Source: CAD feature listing. Evaluate the final solid. Frame: model axes, mm. A direction names the side the tool comes from. Give positions to 0.01 mm unless a question says otherwise; leave off trailing zeros. Loops run counter-clockwise (first coordinate to the right, second up) from the corner with the lowest first, then second, coordinate; pieces in that order, holes last. Notation, with made-up numbers: M 53.5,13.5 L 81.5,13.5 A20 cw 81.5,18.5 Z; hole C 40,-4 d4. An arc over 180 degrees is marked long. Write item = value, one per line.
from build123d import *

# Parameters (mm, degrees)
EXTRUDE_1_DEPTH     = 12
SKETCH_2_R          = 6
EXTRUDE_2_DEPTH     = 9
SKETCH_3_R          = 5.25
EXTRUDE_3_DEPTH     = 1
SKETCH_4_R          = 6
EXTRUDE_4_DEPTH     = 2
CHAMFER_1_SIZE      = 0.5
SKETCH_5_R          = 2
CUT_EXTRUDE_1_DEPTH = 5


with BuildPart() as part:
    # 草图1 → 凸台-拉伸1 (new body)
    with BuildSketch(Plane(origin=(0, 0, 0), x_dir=(1, 0, 0), z_dir=(0, 1, 0))):
        with BuildLine():
            Line((-17.5, 6.09769995), (-6.926984364, 18.843732288))
            ThreePointArc((-6.926984364, 18.843732288), (0, 22.09769995), (6.926984364, 18.843732288))
            Line((6.926984364, 18.843732288), (17.5, 6.09769995))
            Line((17.5, 6.09769995), (17.5, 1.09769995))
            Line((17.5, 1.09769995), (-17.5, 1.09769995))
            Line((-17.5, 1.09769995), (-17.5, 6.09769995))
        make_face()
    extrude(amount=EXTRUDE_1_DEPTH)

    # 草图2 → 凸台-拉伸2 (add)
    with BuildSketch(Plane(origin=(0, 0, 0), x_dir=(1, 0, 0), z_dir=(0, 1, 0))):
        with Locations(Location((0, 13.09769995, 0), (0, 0, 270))):
            Circle(SKETCH_2_R)
    extrude(amount=-EXTRUDE_2_DEPTH)

    # 草图3 → 凸台-拉伸3 (add)
    with BuildSketch(Plane(origin=(0, -9, 0), x_dir=(-1, 0, 0), z_dir=(0, -1, 0))):
        with Locations(Location((0, 13.09769995, 0), (0, 0, 270))):
            Circle(SKETCH_3_R)
    extrude(amount=EXTRUDE_3_DEPTH)

    # 草图4 → 凸台-拉伸4 (add)
    with BuildSketch(Plane(origin=(0, -10, 0), x_dir=(-1, 0, 0), z_dir=(0, -1, 0))):
        with Locations(Location((0, 13.09769995, 0), (0, 0, 270))):
            Circle(SKETCH_4_R)
    extrude(amount=EXTRUDE_4_DEPTH)

    # 倒角1
    chamfer_1_edges = [part.edges().sort_by_distance(p)[0] for p in [
        (0, -12, -19.09769995),
    ]]
    chamfer(chamfer_1_edges, length=CHAMFER_1_SIZE)

    # 草图5 → 切除-拉伸1 (cut)
    with BuildSketch(Plane.XY.offset(-1.09769995)):
        with Locations((-10, 6)):
            Circle(SKETCH_5_R)
        with Locations(Location((10, 6, 0), (0, 0, 180))):
            Circle(SKETCH_5_R)
    extrude(amount=-CUT_EXTRUDE_1_DEPTH, mode=Mode.SUBTRACT)


solid = part.part
1. First-contact query: pin 1 Ø5 at (y, z) = (-4.5, -11.5) entering from -X; pin 2 Ø6 at (y, z) = (5.5, -12) entering from +X; pin 3 Ø3.5 at (x, y) = (10, 6) entering from -Z. Flat tips, straight axial feed; report the tip coordinate or a pass-through.
Derived:
pin_1 = -6
pin_2 = 15.09
pin_3 = -17.25
2. Pull-direction query (Y, two-part tool) for faces 5 (the cylindrical face through (11.6, 7.2, -3.6)), 6 (the cylindrical face through (-0.111, 5.916, -22.097)), 7 (the flat face through (0, -12, -13)); classes: +Y half, -Y half, draft (parallel to the pull), parting line (faces both ways), or undercut.
Derived:
face_5 = undercut
face_6 = draft
face_7 = -Y half
3. Cut plane C-C, the plane x = 10. Return the cut outline in (y, z).
Derived:
outline = M 0,-15.14 L 12,-15.14 L 12,-1.1 L 8,-1.1 L 8,-6.1 L 4,-6.1 L 4,-1.1 L 0,-1.1 Z
4. Cut plane B-B, the plane x = 0. Return the cut outline in (y, z), then the cut area to 3 significant figures.
Derived:
outline = M -12,-18.6 L -11.5,-19.1 L -10,-19.1 L -10,-18.35 L -9,-18.35 L -9,-19.1 L 0,-19.1 L 0,-22.1 L 12,-22.1 L 12,-1.1 L 0,-1.1 L 0,-7.1 L -9,-7.1 L -9,-7.85 L -10,-7.85 L -10,-7.1 L -11.5,-7.1 L -12,-7.6 Z
area = 394 mm²
5. Cut plane D-D, the plane y = -0.75. Return the cut outline in (x, z), then the cut area to 3 significant figures.
Derived:
outline = C 0,-13.1 d12
area = 113 mm²
6. Material intervals for probe 1 along Y at (x, z) = (-10, -2.5); probe 2 along Y at (x, z) = (-9, -12.75); probe 3 along Z at (x, y) = (-5.5, 8.25), sorted ascending. Write a range as from..to.
Derived:
probe_1 = 0..4, 8..12
probe_2 = 0..12
probe_3 = -20.22..-1.1
7. Cut plane A-A, the plane y = 6. Return the cut outline in (x, z).
Derived:
outline = M -17.5,-6.1 L -6.93,-18.84 A9 ccw 6.93,-18.84 L 17.5,-6.1 L 17.5,-1.1 L 12,-1.1 L 12,-6.1 L 8,-6.1 L 8,-1.1 L -8,-1.1 L -8,-6.1 L -12,-6.1 L -12,-1.1 L -17.5,-1.1 Z
8. Reachability of faces 1 (the flat face through (0, 12, -9)), 2 (the flat face through (5, -10, -11)), 3 (the flat face through (10, 6, -6.098)), 4 (the cylindrical face through (2.298, -10.74, -7.555)) from +Z, -Z, +X, -X, +Y, -Y: full face, straight path, thin tool, end or side. Return the list, or none.
Derived:
face_1 = +Z, -Z, +X, -X, +Y
face_2 = none
face_3 = +Z
face_4 = -Y
